from build123d import *

# Parameters (mm, degrees)
F1_DEPTH = 50
F2_DEPTH = 100
F3_R     = 12.5
F4_DEPTH = 50


with BuildPart() as f1:
    # F0 (on Front) → F1 (new body)
    with BuildSketch(Plane.XZ):
        with BuildLine():
            ThreePointArc((-26.841883, 17.345133), (-16.981857, 26.552726), (-13.341859, 39.543118))
            ThreePointArc((-13.341859, 39.543118), (-51.662583, 60.698692), (-49.146524, 16.998513))
            ThreePointArc((-49.146524, 16.998513), (-37.953399, 14.546136), (-26.841883, 17.345133))
        make_face()
    extrude(amount=F1_DEPTH)

    # F0 (on Front) → F2 (join)
    with BuildSketch(Plane.XZ):
        with BuildLine():
            ThreePointArc((-26.841883, 17.345133), (-37.953399, 14.546136), (-49.146524, 16.998513))
            Line((-49.146524, 16.998513), (-49.146524, -48.650906))
            Line((-49.146524, -48.650906), (-26.841883, -48.650906))
            Line((-26.841883, -48.650906), (-26.841883, 17.345133))
        make_face()
    extrude(amount=F2_DEPTH)

    # F3 (on face) → F4 (cut)
    with BuildSketch(Plane.XZ.offset(50)):
        with Locations((-38.341859, 39.543118)):
            Circle(F3_R)
    extrude(amount=-F4_DEPTH, mode=Mode.SUBTRACT)


solid = f1.part
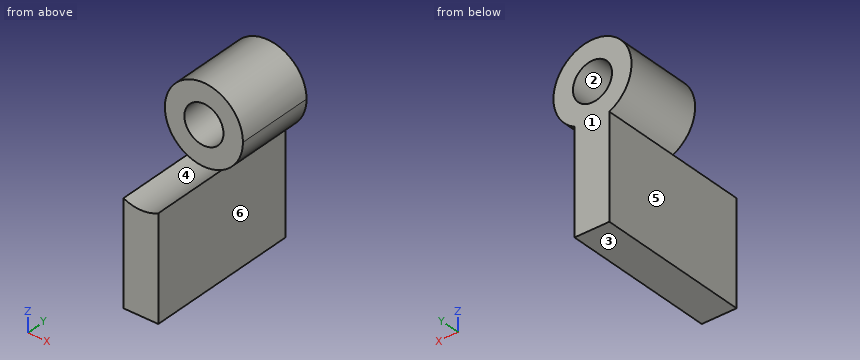
Read the model definition and answer for the solid it produces. Units are mm, in the model's axes. Face numbers are marked on the shaded views. A direction names the side the tool comes from. Round coordinates to 2 decimals unless told otherwise and drop trailing zeros. Loops run counter-clockwise (first coordinate to the right, second up) from the corner with the lowest first, then second, coordinate; pieces in that order, holes last.
Q1. Section B-B on x = -32 is taken. Write down the section's boundary in (y, z), and give its area (3 significant figures).
Q2. Section C-C on z = 2.5 is taken. Write down the section's boundary in (x, y), and give its area (3 significant figures).
Q3. Consider probe 1 along Y at (x, z) = (-23, 38.5); probe 2 along X at (y, z) = (-20.5, -31); probe 3 along Z at (x, y) = (-49, -24). Determine where each line is inside the solid, lowest interval first.
Q4. Which of the six approach directions +Z, -Z, +X, -X, +Y, -Y give full straight-line access (tool end or side, diameter ignored) to the marked faces 4, 5 and 6?
Q5. Section D-D on x = -47.5 is taken. Write down the section's boundary in (y, z).
Q6. Determine the mould class of the marked faces 1, 2 and 3 for opening direction Z: released by +Z, released by -Z, zero draft, split by the parting line, or undercut.
Q7. Each of these flat-tipped pins is pushed along its axis until it touches: pin 1 (6 mm diameter, centred on y = -58.5, z = 17.5, fed in from -X); pin 2 (8 mm diameter, centred on x = -19.5, z = -13.5, fed in from +Y); pin 3 (1 mm diameter, centred on x = -30, z = -8, fed in from +Y); pin 4 (1 mm diameter, centred on x = -55.5, y = -18, fed in from -Z). Where does it stop, or does it pass through?
Q8. Section A-A on y = -16.5 is taken. Write down the section's boundary in (x, z).
Output:
1. outline: (-100, -48.65) - (0, -48.65) - (0, 28.77) - (-50, 28.77) - (-50, 15.36) - (-100, 15.36) - close; (-50, 50.31) - (0, 50.31) - (0, 63.73) - (-50, 63.73) - close
1. area: 7,740 mm2
2. outline: (-49.15, -100) - (-26.84, -100) - (-26.84, 0) - (-49.15, 0) - close
2. area: 2,230 mm2
3. probe 1: y = -50 to 0
3. probe 2: x = -49.15 to -26.84
3. probe 3: z = -48.65 to 33.01, 46.07 to 62.16
4. face 4: +Z, -Y
4. face 5: -Z, -X, +Y, -Y
4. face 6: -Z, +X, +Y, -Y
5. outline: (-100, -48.65) - (0, -48.65) - (0, 31.04) - (-50, 31.04) - (-50, 16.28) - (-100, 16.28) - close; (-50, 48.05) - (0, 48.05) - (0, 62.81) - (-50, 62.81) - close
6. face 1: zero draft
6. face 2: undercut
6. face 3: released by -Z
7. pin 1: stops at x = -49.15
7. pin 2: passes through
7. pin 3: stops at y = 0
7. pin 4: stops at z = 20.9
8. outline: (-49.15, -48.65) - (-26.84, -48.65) - (-26.84, 17.35) arc R25 ccw to (-13.34, 39.54) arc R25 ccw (long way) to (-49.15, 17) - close; hole circle Ø25 at (-38.34, 39.54)
